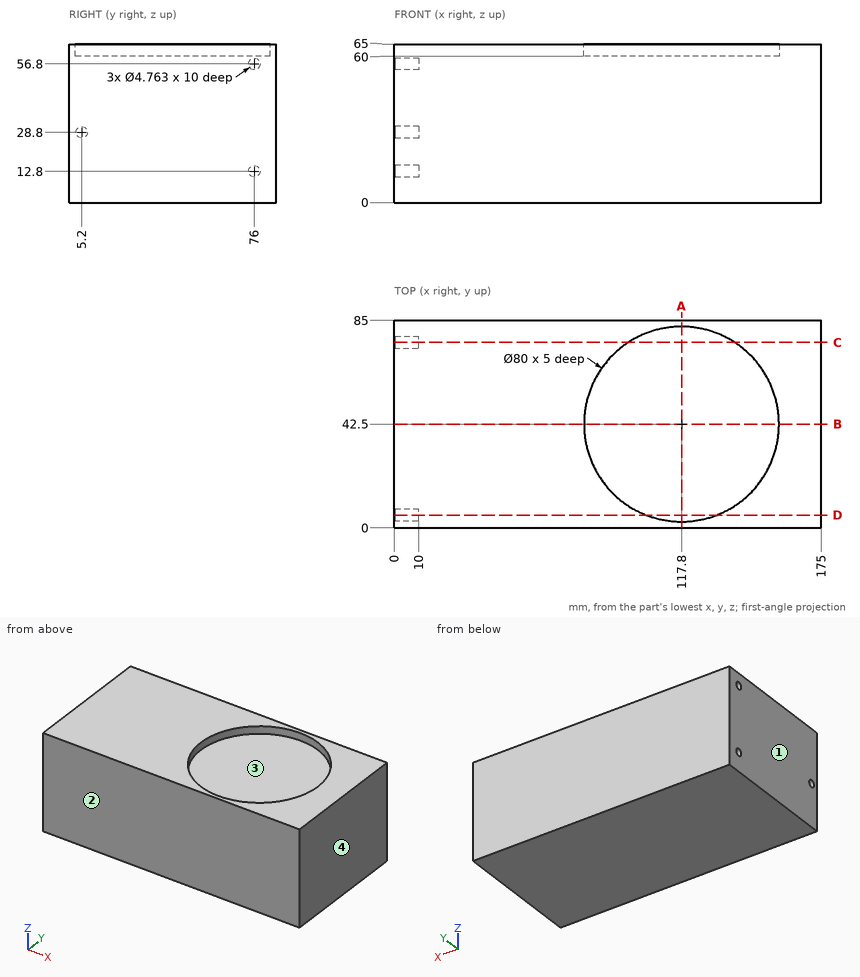
Here's the drawing with two shaded views (mm, measured from the low corner). I have some questions. Coordinates: 2 decimals unless noted, no trailing zeros. Write each loop counter-clockwise with the first axis right and the second up, starting at its lowest first coordinate (ties: lowest second). Pieces come first, ordered by that corner, then holes. Notation, with made-up numbers: (1.25, 29) - (22.25, 29) arc R33 ccw to (22.25, 57) - close; hole circle Ø11 at (-18.75, 46). An arc over 180 degrees is marked (long way). Return JSON: item names as keys, results as strings.
Q1. If we section it at C-C (y = 76): Please give me the cut outline in (x, z), then the cut area to 3 significant figures.
Computed values:
{"outline": "(0, 0) - (175, 0) - (175, 65) - (139.66, 65) - (139.66, 60) - (95.94, 60) - (95.94, 65) - (0, 65) - (0, 59.18) - (10, 59.18) - (10, 54.42) - (0, 54.42) - (0, 15.18) - (10, 15.18) - (10, 10.42) - (0, 10.42) - close", "area": "11,100 mm2"}
Q2. I'm going to push a flat-ended pin straight in: pin 1 Ø4 at (y, z) = (76, 56.8) entering from -X. Where does the tip first touch, or does it pass through?
Computed values:
{"pin 1": "stops at x = 10"}
Q3. Thinking about a two-plate mould opening in X: for the marked faces 1, 2, 3 and 4, which applies, +X half, -X half, draft (parallel to the pull), parting line (faces both ways), or undercut?
Computed values:
{"face 1": "-X half", "face 2": "draft", "face 3": "undercut", "face 4": "+X half"}
Q4. If we section it at D-D (y = 5.2): Please give me the cut outline in (x, z), then the cut area to 3 significant figures.
Computed values:
{"outline": "(0, 0) - (175, 0) - (175, 65) - (132.25, 65) - (132.25, 60) - (103.35, 60) - (103.35, 65) - (0, 65) - (0, 31.18) - (10, 31.18) - (10, 26.42) - (0, 26.42) - close", "area": "11,200 mm2"}
Q5. Please list where these lines run through material, in increasing order: L1, parallel to Z at x = 5, y = 76; L2, parallel to Y at x = 117, z = 61; L3, parallel to Z at x = 134, y = 57. Write a range as from..to.
Computed values:
{"L1": "z = 0..10.42, 15.18..54.42, 59.18..65", "L2": "y = 0..2.51, 82.49..85", "L3": "z = 0..60"}
Q6. If we section it at A-A (x = 117.8): Please give me the cut outline in (y, z).
Computed values:
{"outline": "(0, 0) - (85, 0) - (85, 65) - (82.5, 65) - (82.5, 60) - (2.5, 60) - (2.5, 65) - (0, 65) - close"}
Q7. If we section it at B-B (y = 42.5): Please give me the cut outline in (x, z).
Computed values:
{"outline": "(0, 0) - (175, 0) - (175, 65) - (157.8, 65) - (157.8, 60) - (77.8, 60) - (77.8, 65) - (0, 65) - close"}
